Here's how the part is built. I have some questions about the finished solid (model axes, mm). A direction names the side the tool comes from. Coordinates: 2 decimals unless noted, no trailing zeros. Write each loop counter-clockwise with the first axis right and the second up, starting at its lowest first coordinate (ties: lowest second). Pieces come first, ordered by that corner, then holes.
Item 1: If I drill on line 1 (Y direction, x = 67, z = -15), over which ranges is the centre line in solid material (lowest first)?
Item 2: If we section it at B-B (z = -12): Please give me the cut outline in (x, y).
Item 3: I'm going to push a flat-ended pin straight in: pin 1 Ø3 at (x, z) = (122.5, -15.5) entering from +Y. Where does the tip first touch, or does it pass through?
Item 4: If we section it at C-C (x = 19): Please give me the cut outline in (y, z), then the cut area to 3 significant figures.
Item 5: If we section it at A-A (x = 33.4): Please give me the cut outline in (y, z), then the cut area to 3 significant figures.
Item 6: For faces 1 (the face through (68, 0, -17)), 2 (the face through (40.554, 148.103, -19.253)), which set-ups out of +Z, -Z, +X, -X, +Y, -Y let a thin tool reach every point of the face, with its end or its side?
Item 7: We'd pull the mould along X, two halves only. Please class faces 3 (the face through (137.7, 70, -17)), 4 (the face through (68, 70, -34)), 5 (the face through (0, 70, -17)), 6 (the face through (111.454, 148.103, -19.253)): +X half, -X half, draft (parallel to the pull), parting line (faces both ways), or undercut.
from build123d import *

# Parameters (mm, degrees)
SKETCH1_W           = 137.7
SKETCH1_H           = 34
BOSS_EXTRUDE1_DEPTH = 141.3
SKETCH2_R           = 7.5
BOSS_EXTRUDE2_DEPTH = 13.8


with BuildPart() as part:
    # Sketch1 → Boss-Extrude1 (new body)
    with BuildSketch(Plane(origin=(0, 0, 0), x_dir=(1, 0, 0), z_dir=(0, 1, 0))):
        with Locations((68.85, 17)):
            Rectangle(SKETCH1_W, SKETCH1_H)
    extrude(amount=BOSS_EXTRUDE1_DEPTH)

    # Sketch2 → Boss-Extrude2 (add)
    with BuildSketch(Plane(origin=(0, 141.3, 0), x_dir=(1, 0, 0), z_dir=(0, 1, 0))):
        with Locations((33.4, 17)):
            Circle(SKETCH2_R)
        with Locations((104.3, 17)):
            Circle(SKETCH2_R)
    extrude(amount=BOSS_EXTRUDE2_DEPTH)


solid = part.part
Answer list:
1. line 1: y = 0 to 141.3
2. outline: (0, 0) - (137.7, 0) - (137.7, 141.3) - (109.89, 141.3) - (109.89, 155.1) - (98.71, 155.1) - (98.71, 141.3) - (38.99, 141.3) - (38.99, 155.1) - (27.81, 155.1) - (27.81, 141.3) - (0, 141.3) - close
3. pin 1: stops at y = 141.3
4. outline: (0, -34) - (141.3, -34) - (141.3, 0) - (0, 0) - close
4. area: 4,800 mm2
5. outline: (0, -34) - (141.3, -34) - (141.3, -24.5) - (155.1, -24.5) - (155.1, -9.5) - (141.3, -9.5) - (141.3, 0) - (0, 0) - close
5. area: 5,010 mm2
6. face 1: +Z, -Z, +X, -X, -Y
6. face 2: +Y
7. face 3: +X half
7. face 4: draft
7. face 5: -X half
7. face 6: undercut
